```python
from build123d import *

# Parameters (mm, degrees)
PAD_DEPTH    = 10
SKETCH001_W  = 10
SKETCH001_H  = 40
PAD001_DEPTH = 30
SKETCH002_W  = 20
SKETCH002_H  = 40
PAD002_DEPTH = 10
PAD003_DEPTH = 30
POCKET_DEPTH = 10


with BuildPart() as part:
    # Sketch → Pad (new body)
    with BuildSketch(Plane.XY):
        with BuildLine():
            Line((37.5, -20), (37.5, 20))
            Line((37.5, 20), (-37.5, 20))
            ThreePointArc((-37.5, 20), (-57.5, 0), (-37.5, -20))
            Line((-37.5, -20), (37.5, -20))
        make_face()
    extrude(amount=PAD_DEPTH)

    # Sketch001 (on Face6 of Pad) → Pad001 (join)
    with BuildSketch(Plane.XY.offset(10)):
        with Locations((32.5, 0)):
            Rectangle(SKETCH001_W, SKETCH001_H)
    extrude(amount=PAD001_DEPTH)

    # Sketch002 (on Face5 of Pad001) → Pad002 (join)
    with BuildSketch(Plane.XY.offset(40)):
        with Locations((27.5, 0)):
            Rectangle(SKETCH002_W, SKETCH002_H)
    extrude(amount=PAD002_DEPTH)

    # Sketch003 (on Face3 of Pad002) → Pad003 (join)
    with BuildSketch(Plane.XY.offset(10)):
        with BuildLine():
            Line((-56.864917, 5), (27.5, 5))
            Line((27.5, 5), (27.5, -5))
            Line((-56.864917, -5), (27.5, -5))
            ThreePointArc((-56.864917, 5), (-57.5, 0), (-56.864917, -5))
        make_face()
    extrude(amount=PAD003_DEPTH)

    # Sketch004 (on Face15 of Pad003) → Pocket (cut)
    with BuildSketch(Plane.XZ.offset(5)):
        Polygon((-57.5, 10), (17.5, 40), (-57.5, 40), align=None)
    extrude(amount=-POCKET_DEPTH, mode=Mode.SUBTRACT)


solid = part.part
```
Part model, mm, in its own coordinate system. A direction names the side the tool comes from. Round coordinates to 2 decimals unless told otherwise and drop trailing zeros. Write each loop counter-clockwise with the first axis right and the second up, starting at its lowest first coordinate (ties: lowest second). Pieces come first, ordered by that corner, then holes.
Item 1: Probe L1, parallel to Z at x = 22.5, y = 6; L2, parallel to X at y = -8, z = 32; L3, parallel to X at y = 8.5, z = 40.5. List the from-to ranges inside material, lowest first.
Results:
L1: z = 0 to 10, 40 to 50
L2: x = 27.5 to 37.5
L3: x = 17.5 to 37.5
Item 2: Cut at B-B, the plane z = 12. Give the cut face in (x, y).
Results:
outline: (-52.5, -5) - (27.5, -5) - (27.5, -20) - (37.5, -20) - (37.5, 20) - (27.5, 20) - (27.5, 5) - (-52.5, 5) - close
Item 3: Cut at C-C, the plane y = 1. Give the cut face in (x, z).
Results:
outline: (-57.47, 0) - (37.5, 0) - (37.5, 50) - (17.5, 50) - (17.5, 40) - (-57.47, 10.01) - close
Item 4: Cut at D-D, the plane y = -3.5. Give the cut face in (x, z), plus the area to 3 significant figures.
Results:
outline: (-57.19, 0) - (37.5, 0) - (37.5, 50) - (17.5, 50) - (17.5, 40) - (-57.19, 10.12) - close
area: 2,870 mm2
Item 5: Which spindle directions (+Z, -Z, +X, -X, +Y, -Y) get a long thin tool onto all of the face, cutting with end or side? Do faces 1 (the flat face through (27.5, -13, 25)), 2 (the flat face through (-6, 5, 21)), 3 (the flat face through (17.5, 0, 45)), 4 (the flat face through (14, -20, 8)). Say none if no direction does.
Results:
face 1: -X, -Y
face 2: -X, +Y
face 3: +Z, -X, +Y, -Y
face 4: +Z, -Z, +X, -X, -Y
Item 6: Cut at A-A, the plane x = -8.5. Give the cut face in (y, z), plus the area to 3 significant figures.
Results:
outline: (-20, 0) - (20, 0) - (20, 10) - (5, 10) - (5, 29.6) - (-5, 29.6) - (-5, 10) - (-20, 10) - close
area: 596 mm2
Item 7: Drop flat-ended pins along their axis: pin 1 Ø7.5 at (x, y) = (-5, -14) entering from +Z; pin 2 Ø24 at (x, z) = (-30.5, 29.5) entering from +Y; pin 3 Ø1 at (x, z) = (1, 25) entering from -Y. Give the stop position or say it passes through.
Results:
pin 1: stops at z = 10
pin 2: stops at y = 5
pin 3: stops at y = -5
